from build123d import *

# Parameters (mm, degrees)
F0_W     = 76.2
F0_H     = 76.2
F1_DEPTH = 5.08
F3_DEPTH = 76.2
F4_ANGLE = -90


with BuildPart() as f1:
    # F0 (on Front) → F1 (new body)
    with BuildSketch(Plane.XZ):
        with Locations((38.1, 38.1)):
            Rectangle(F0_W, F0_H)
    extrude(amount=-F1_DEPTH)

    # F2 (on face) → F3 (join)
    with BuildSketch(Plane(origin=(0, 0, 0), x_dir=(1, 0, 0), z_dir=(0, 0, -1))):
        with BuildLine():
            ThreePointArc((56.0605122421, 0), (52.3943380328, 1.1652467111), (50.0736748281, 4.2333333333))
            ThreePointArc((50.0736748281, 4.2333333333), (38.1, 12.7), (26.1263251719, 4.2333333333))
            ThreePointArc((26.1263251719, 4.2333333333), (23.8056619672, 1.1652467111), (20.1394877579, 0))
            Line((20.1394877579, 0), (56.0605122421, 0))
        make_face()
    extrude(amount=-F3_DEPTH)


with BuildPart() as f1_1:
    # F4: moved
    add(f1.part.rotate(Axis((10.0697438789, 0, 0), (1, 0, 0)), F4_ANGLE))


solid = f1_1.part
CAD build for the part. Positions are in the model's coordinates, mm. A direction names the side the tool comes from. Round coordinates to 2 decimals unless told otherwise and drop trailing zeros. Write each loop counter-clockwise with the first axis right and the second up, starting at its lowest first coordinate (ties: lowest second). Pieces come first, ordered by that corner, then holes. Notation, with made-up numbers: (71.25, -23.5) -> (122.25, -23.5) arc R21 cw to (122.25, -2.5) -> close; hole circle Ø9 at (33.25, 48.5). An arc over 180 degrees is marked (long way). Answer as a JSON object with one key per item and string values.
(1) Band-saw the part on C-C, the plane z = 11.5. List the corners of the cut face in (x, y), then the cut area to 3 significant figures.
Reported:
{"outline": "(32.71, 0) -> (43.49, 0) -> (43.49, 76.2) -> (32.71, 76.2) -> close", "area": "821 mm^2"}
(2) Pin check, flat tips, straight feed: P1, Ø8, axis at y = 9.5, z = 10.5, coming from the +X side; P2, Ø4, axis at y = 11.5, z = 10, coming from the -X side; P3, Ø8, axis at x = 66, y = 12, coming from the +Z side. Stop position of each tip, or through.
Reported:
{"P1": "stops at x = 49.01", "P2": "stops at x = 28.24", "P3": "stops at z = 0"}
(3) Which spindle directions (+Z, -Z, +X, -X, +Y, -Y) get a long thin tool onto all of the face, cutting with end or side? Do faces 1 (the face through (10, 39, 0)), 2 (the face through (38, 76.2, 0)), 3 (the face through (66, 39, 0)). Say none if no direction does.
Reported:
{"face 1": "+Z, -X, +Y, -Y", "face 2": "+Z, -Z, +X, -X, +Y", "face 3": "+Z, +X, +Y, -Y"}
(4) Probe probe 1 along Z at (x, y) = (67, 39.5); probe 2 along X at (y, z) = (32, 0.5); probe 3 along X at (y, z) = (45.5, 1.25). List the from-to ranges inside material, lowest first. Write a range as [from, to].
Reported:
{"probe 1": "z = [-5.08, 0]", "probe 2": "x = [22.61, 53.59]", "probe 3": "x = [23.92, 52.28]"}
(5) Band-saw the part on A-A, the plane y = 40.5. List the corners of the cut face in (x, z).
Reported:
{"outline": "(0, -5.08) -> (76.2, -5.08) -> (76.2, 0) -> (56.06, 0) arc R6.35 cw to (50.07, 4.23) arc R12.7 ccw to (26.13, 4.23) arc R6.35 cw to (20.14, 0) -> (0, 0) -> close"}
(6) Band-saw the part on B-B, the plane x = 7.5. List the corners of the cut face in (y, z).
Reported:
{"outline": "(0, -5.08) -> (76.2, -5.08) -> (76.2, 0) -> (0, 0) -> close"}
